Autodesk Inventor part; units mm, degrees
ref_plane "spring_washer_to_bolt_XY" through (0, 0, 0) normal (1, 0, 0) x (0, 0, -1)
ref_plane "spring_washer_to_bolt_YZ" through (0, 0, 0) normal (0, 0, -1) x (0, 1, 0)
ref_plane "spring_washer_to_bolt_ZX" through (0, 0, 0) normal (0, 1, 0) x (1, 0, 0)
sketch "Sketch_1" plane through (0, 0, 0) normal (0, 0, 1) x (1, 0, 0)
  line L0 (0.27, 0) -> (-0.27, 0)
  line L1 (-0.27, 0) -> (-0.27, 4.25)
  line L2 (-0.27, 4.25) -> (0.27, 4.25)
  line L3 (0.27, 4.25) -> (0.27, 0)
  line L4 (0.27, 0) -> (-0.27, 0)
revolve "Revolution1" add sketch "Sketch_1" angle 180 about axis through (0.27, 0, 0) along (-1, 0, 0)
sketch "Sketch_2" plane through (0, 0, 0) normal (0, 0, 1) x (1, 0, 0)
  line L0 (0.27, -0.0476) -> (-0.27, 0.0476)
  line L1 (-0.27, 0.0476) -> (-0.27, 4.25)
  line L2 (-0.27, 4.25) -> (0.27, 4.25)
  line L3 (0.27, 4.25) -> (0.27, -0.0476)
  line L4 (0.27, -0.0476) -> (-0.27, 0.0476)
revolve "Revolution2" add sketch "Sketch_2" angle 90 about axis through (0.27, -0.0476, 0) along (0.9848078, -0.1736482, 0)
sketch "Sketch_3" plane through (0, 0, 0) normal (0, 0, 1) x (1, 0, 0)
  line L0 (-0.27, 0.0476) -> (0.27, -0.0476)
  line L1 (0.27, -0.0476) -> (0.27, -4.25)
  line L2 (0.27, -4.25) -> (-0.27, -4.25)
  line L3 (-0.27, -4.25) -> (-0.27, 0.0476)
  line L4 (-0.27, 0.0476) -> (0.27, -0.0476)
revolve "Revolution3" add sketch "Sketch_3" angle 90 about axis through (-0.27, 0.0476, 0) along (-0.9848078, 0.1736482, 0)
sketch "Sketch_4" plane through (0, 0, 0) normal (1, 0, 0) x (0, 1, 0)
  line L0 (-1.0625, 4.25) -> (-1.0625, 2.263)
  arc A0 (-1.0625, 2.263) -> (1.0625, 2.263) centre (0, 0) ccw
  line L1 (1.0625, 2.263) -> (1.0625, 4.25)
  line L2 (1.0625, 4.25) -> (-1.0625, 4.25)
extrude "Extrusion1" cut sketch "Sketch_4" along normal mid plane 17
ref_plane "spring_washer_to_bolt_XY" through (0, 0, 0) normal (1, 0, 0) x (0, 0, -1)
ref_plane "spring_washer_to_bolt_YZ" through (0, 0, 0) normal (0, 0, -1) x (0, 1, 0)
ref_plane "spring_washer_to_bolt_ZX" through (0, 0, 0) normal (0, 1, 0) x (1, 0, 0)
properties part number "Washer-Spring5"
CAD build for the part. Positions are in the model's coordinates, mm. A direction names the side the tool comes from. Give positions to 0.01 mm unless a question says otherwise; leave off trailing zeros. Order: outer loops, then holes, each group sorted by start corner. A loop starts at its lowest first (then second) coordinate and runs counter-clockwise, first axis right, second up. Notation, with made-up numbers: (10.25, -2.5) - (51.25, -2.5) arc R10 ccw to (51.25, 11.5) - close; hole circle Ø8 at (57.5, -23.5). An arc over 180 degrees is marked (long way). Write each question's results on one line, items separated by ' | '.
1. 3-axis set-ups, long thin cutter, end or side, ignore diameter. For faces 4 (the face through (-0.39, 2.5, 1.96)), 5 (the face through (-0.15, -2.49, 1.99)), 6 (the face through (-0.27, 0, -3)): which of +Z, -Z, +X, -X, +Y, -Y reach the whole face in a straight line?
Calculated:
face 4: -Z, -X, +Y | face 5: +Z, -X | face 6: -Z, -X, +Y, -Y
2. Pull direction Y, two halves, no side cores. Call faces 1 (the face through (0.21, -3.37, 2.58)), 2 (the face through (0.15, 2.49, 1.99)), 3 (the face through (0.27, 0, -3)): released by +Y, released by -Y, zero draft, split by the parting line, or undercut.
Calculated:
face 1: released by -Y | face 2: undercut | face 3: zero draft
3. Saw through at A-A on z = -2. List the corners of the cut face in (x, y), and give its area (3 significant figures).
Calculated:
outline: (-0.27, -3.75) - (0.27, -3.75) - (0.27, -1.5) - (-0.27, -1.5) - close; (-0.27, 1.5) - (0.27, 1.5) - (0.27, 3.75) - (-0.27, 3.75) - close | area: 2.43 mm2
4. Pin check, flat tips, straight feed: pin 1 (1.3 mm diameter, centred on y = 0, z = -3, fed in from +X); pin 2 (0.9 mm diameter, centred on x = 0.5, z = 3.5, fed in from +Y); pin 3 (1.3 mm diameter, centred on y = 0, z = -2.5, fed in from -X). Stop position of each tip, or through.
Calculated:
pin 1: stops at x = 0.27 | pin 2: stops at y = -1.06 | pin 3: stops at x = -0.27
5. Probe L1, parallel to Y at x = 0, z = 0; L2, parallel to X at y = 1, z = -3.25; L3, parallel to Z at x = 0.05, y = 0. List the from-to ranges inside material, lowest first. Write a range as from..to.
Calculated:
L1: y = -4.25..-2.5, 2.5..4.25 | L2: x = -0.27..0.27 | L3: z = -4.25..-2.5
6. Saw through at B-B on y = 0. List the corners of the cut face in (x, z), and give its area (3 significant figures).
Calculated:
outline: (-0.27, -4.25) - (0.27, -4.25) - (0.27, -2.5) - (-0.27, -2.5) - close | area: 0.945 mm2
7. Saw through at C-C on z = -3.5. List the corners of the cut face in (x, y).
Calculated:
outline: (-0.27, -2.41) - (0.27, -2.41) - (0.27, 2.41) - (-0.27, 2.41) - close
